Design review of the part built by this model. Coordinates are the model's own, in mm. Face numbers are marked on the shaded views. A direction names the side the tool comes from. Round coordinates to 2 decimals unless told otherwise and drop trailing zeros. Loops run counter-clockwise (first coordinate to the right, second up) from the corner with the lowest first, then second, coordinate; pieces in that order, holes last. Notation, with made-up numbers: (-19, -12.75) - (13, -12.75) arc R24 cw to (13, -2.75) - close; hole circle Ø1 at (-23.5, 43.25). An arc over 180 degrees is marked (long way). Use one line per item in the form item = value. Start each with the question number.
(1) Wall thickness on probe 1 along X at (y, z) = (1.5, 22.5); probe 2 along X at (y, z) = (6, 16); probe 3 along X at (y, z) = (-4, 27.5): over which ranges is each line inside the solid? List them lowest first. Write a range as [from, to].
(2) We need section A-A, the plane y = -2.75. Write out the cut boundary in (x, z).
(3) We need section C-C, the plane x = 6.5. Write out the cut boundary in (y, z).
(4) We need section B-B, the plane z = 20.5. Write out the cut boundary in (x, y), then the cut area to 3 significant figures.
(5) Machinability: for the marked faces 1, 2, 3, 4 and 5, which of the approach directions +Z, -Z, +X, -X, +Y, -Y give a long, thin tool a straight path to every point of the face, cutting with its end or side? Answer none if there is none.
(6) For pin 1 (1 mm diameter, centred on x = -6.5, z = 22.5, fed in from -Y); pin 2 (5 mm diameter, centred on x = -28.5, y = -5, fed in from -Z); pin 3 (2 mm diameter, centred on y = 4, z = 23, fed in from +X); pin 4 (5.5 mm diameter, centred on x = -18.5, y = 3.5, fed in from +Z), all flat-tipped, find the tip position at first contact; note any pin that passes through.
(7) We need section D-D, the plane x = -7. Write out the cut boundary in (y, z).
(8) The part is to be moulded in two halves that separate along Y. For the marked faces 6, 7, 8 and 9, say which applies: released by +Y, released by -Y, zero draft, split by the parting line, or undercut.
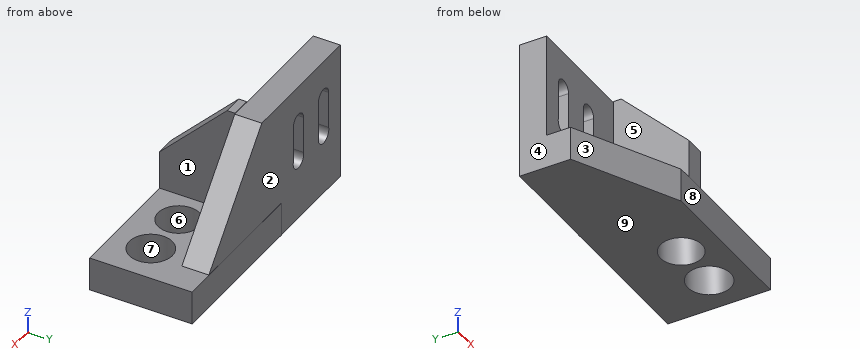
from build123d import *

# Parameters (mm, degrees)
F0_W      = 35.6949009001
F0_H      = 36.5447811782
F1_DEPTH  = 7.112
F2_W      = 26.9532920793
F2_H      = 13.2338248659
F3_DEPTH  = 8.89
F4_W      = 5.3117033094
F4_H      = 27.8393924236
F5_DEPTH  = 19.812
F6_SIZE   = 17.78
F8_DEPTH  = 25.4
F9_R      = 5.4567571196
F9_R_2    = 5.6687450147
F10_DEPTH = 25.4


with BuildPart() as f1:
    # F0 (on Front) → F1 (new body)
    with BuildSketch(Plane.XZ):
        with Locations((-17.8474504501, 18.2723905891)):
            Rectangle(F0_W, F0_H)
        Polygon((0, 36.5447811782), (0, 0), (31.8097434938, 0), align=None)
    extrude(amount=-F1_DEPTH)

    # F2 (on Top) → F3 (join)
    with BuildSketch(Plane.XY):
        Polygon((31.8097434938, 7.1632624604), (-8.7416088209, 7.1632624604), (-8.7416088209, 6.9204405881), (-8.7416088209, -6.3133842777), (-8.7416088209, -19.7900310159), (31.8097434938, -19.7900310159), align=None)
        with Locations((-22.2182548605, 0.3035281552)):
            Rectangle(F2_W, F2_H)
        Polygon((-8.7416088209, -19.7900310159), (-8.7416088209, -6.3133842777), (-35.6949009001, -6.3133842777), align=None)
    extrude(amount=F3_DEPTH)

    # F4 (on Front) → F5 (join)
    with BuildSketch(Plane.XZ):
        with Locations((-2.6558516547, 22.8818580508)):
            Rectangle(F4_W, F4_H)
    extrude(amount=F5_DEPTH)

    # F6
    f6_edges = [f1.edges().sort_by_distance(p)[0] for p in [
        (-2.655852, -19.812, 36.801554),
    ]]
    chamfer(f6_edges, length=F6_SIZE)

    # F7 (on Front) → F8 (cut)
    with BuildSketch(Plane.XZ):
        with BuildLine():
            ThreePointArc((-25.7391817868, 26.5890602022), (-28.0459942296, 28.8958726451), (-30.3528066725, 26.5890602022))
            Line((-30.3528066725, 26.5890602022), (-30.3528066725, 16.8761610985))
            ThreePointArc((-30.3528066725, 16.8761610985), (-28.0459942296, 13.8837524755), (-25.7391817868, 16.8761610985))
            Line((-25.7391817868, 16.8761610985), (-25.7391817868, 26.5890602022))
        make_face()
        with BuildLine():
            Line((-18.9401526004, 26.5890602022), (-18.9401526004, 16.8761610985))
            ThreePointArc((-18.9401526004, 16.8761610985), (-16.6333387606, 13.93419969), (-14.3265249208, 16.8761610985))
            Line((-14.3265249208, 16.8761610985), (-14.3265249208, 26.5890602022))
            ThreePointArc((-14.3265249208, 26.5890602022), (-16.6333387606, 28.8958740421), (-18.9401526004, 26.5890602022))
        make_face()
    extrude(amount=-F8_DEPTH, mode=Mode.SUBTRACT)

    # F9 (on face) → F10 (cut)
    with BuildSketch(Plane.XY.offset(8.89)):
        with Locations((8.4987860173, -9.8343091086)):
            Circle(F9_R)
        with Locations((21.6111987829, -9.5914872363)):
            Circle(F9_R_2)
    extrude(amount=-F10_DEPTH, mode=Mode.SUBTRACT)


solid = f1.part
Data:
q1.probe_1 = [-35.69, -30.35], [-25.74, -18.94], [-14.33, 12.23]
q1.probe_2 = [-35.69, -30.42], [-25.68, -18.99], [-14.28, 17.88]
q1.probe_3 = [-5.31, 0]
q2.outline = (-35.69, 0) - (31.81, 0) - (31.81, 8.89) - (-35.69, 8.89) - close; (-5.31, 8.96) - (0, 8.96) - (0, 36.08) - (-5.31, 36.08) - close
q3.outline = (-19.79, 0) - (-14.91, 0) - (-14.91, 8.89) - (-19.79, 8.89) - close; (-4.76, 0) - (7.16, 0) - (7.16, 8.89) - (7.11, 8.89) - (7.11, 29.08) - (0, 29.08) - (0, 8.89) - (-4.76, 8.89) - close
q4.outline = (-35.69, 0) - (-30.35, 0) - (-30.35, 7.11) - (-35.69, 7.11) - close; (-25.74, 0) - (-18.94, 0) - (-18.94, 7.11) - (-25.74, 7.11) - close; (-14.33, 0) - (-5.31, 0) - (-5.31, -18.33) - (0, -18.33) - (0, 0) - (13.97, 0) - (13.97, 7.11) - (-14.33, 7.11) - close
q4.area = 385 mm^2
q5.face_1 = +Z, +X, -Y
q5.face_2 = +Z, -X, +Y
q5.face_3 = +Z, -Z, -X, -Y
q5.face_4 = +Z, -Z, -X, +Y, -Y
q5.face_5 = +Z, -X, -Y
q6.pin_1 = 0
q6.pin_2 = 0
q6.pin_3 = 12.66
q6.pin_4 = 36.54
q7.outline = (-19.79, 0) - (7.16, 0) - (7.16, 8.89) - (7.11, 8.89) - (7.11, 36.54) - (0, 36.54) - (0, 8.89) - (-19.79, 8.89) - close
q8.face_6 = undercut
q8.face_7 = undercut
q8.face_8 = released by -Y
q8.face_9 = zero draft
